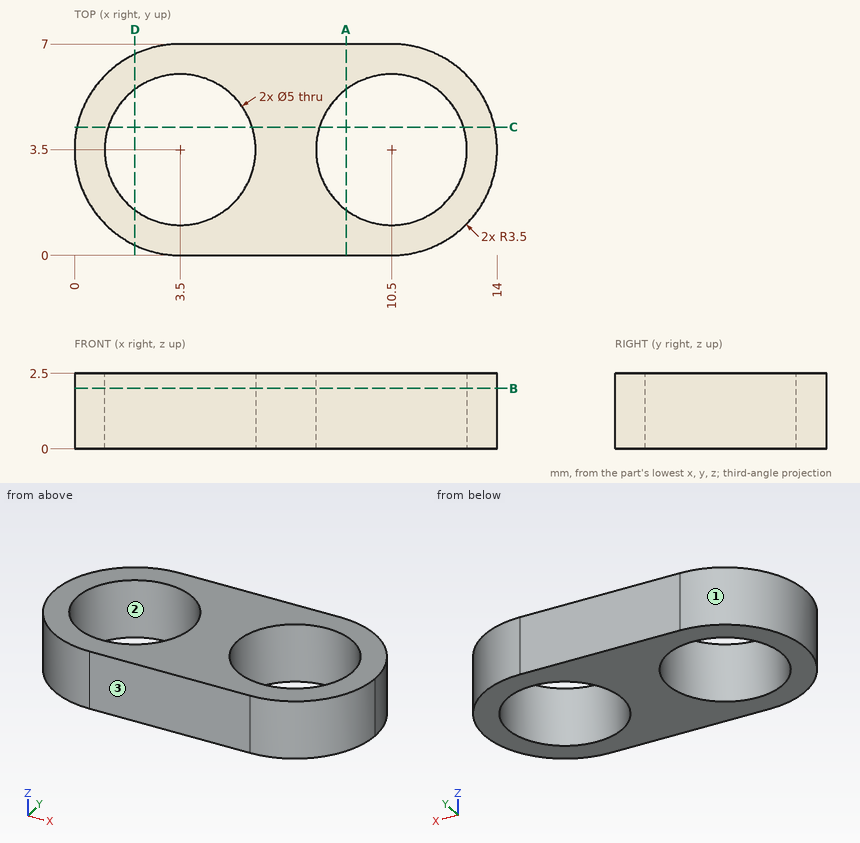
Source: three-view drawing plus pictorial views. Frame: mm from the lowest corner of the part. Give positions to 0.01 mm unless a question says otherwise; leave off trailing zeros. Write each loop counter-clockwise with the first axis right and the second up, starting at its lowest first coordinate (ties: lowest second). Pieces come first, ordered by that corner, then holes. Notation, with made-up numbers: (-40, 39) - (-17, 39) arc R12 cw to (-17, 62) - close; hole circle Ø5 at (-4.75, 12.25). An arc over 180 degrees is marked (long way). Write item = value, one per line. Start each with the question number.
1. Mould query, pull axis X, two halves, no side actions, for the marked faces 1, 2 and 3. Classes: released by +X, released by -X, zero draft, split by the parting line, or undercut.
2. Ray query, L1, parallel to X at y = 5, z = 0.85; L2, parallel to X at y = 3.25, z = 1.2; L3, parallel to Y at x = 3.5, z = 1.85. Return the intervals inside material, ascending.
3. Section query D-D, the plane x = 2. Output: boundary loops of the cut face in (y, z).
4. Section query A-A, the plane x = 9. Output: boundary loops of the cut face in (y, z).
5. First-contact query: pin 1 Ø4 at (x, y) = (2.5, 2) entering from -Z; pin 2 Ø1.5 at (y, z) = (1, 2) entering from +X. Flat tips, straight axial feed; report the tip coordinate or a pass-through.
6. Section query B-B, the plane z = 2. Output: boundary loops of the cut face in (x, y), then the cut area to 3 significant figures.
7. Section query C-C, the plane y = 4.25. Output: boundary loops of the cut face in (x, z), then the cut area to 3 significant figures.
Check sheet entries:
q1.face_1 = released by -X
q1.face_2 = undercut
q1.face_3 = zero draft
q2.L1 = 0.34 to 1.5, 5.5 to 8.5, 12.5 to 13.66
q2.L2 = 0.01 to 1.01, 5.99 to 8.01, 12.99 to 13.99
q2.L3 = 0 to 1, 6 to 7
q3.outline = (0.34, 0) - (1.5, 0) - (1.5, 2.5) - (0.34, 2.5) - close; (5.5, 0) - (6.66, 0) - (6.66, 2.5) - (5.5, 2.5) - close
q4.outline = (0, 0) - (1.5, 0) - (1.5, 2.5) - (0, 2.5) - close; (5.5, 0) - (7, 0) - (7, 2.5) - (5.5, 2.5) - close
q5.pin_1 = 0
q5.pin_2 = 13.53
q6.outline = (3.5, 0) - (10.5, 0) arc R3.5 ccw to (10.5, 7) - (3.5, 7) arc R3.5 ccw to start; hole circle Ø5 at (3.5, 3.5); hole circle Ø5 at (10.5, 3.5)
q6.area = 48.2 mm2
q7.outline = (0.08, 0) - (1.12, 0) - (1.12, 2.5) - (0.08, 2.5) - close; (5.88, 0) - (8.12, 0) - (8.12, 2.5) - (5.88, 2.5) - close; (12.88, 0) - (13.92, 0) - (13.92, 2.5) - (12.88, 2.5) - close
q7.area = 10.7 mm2
